Can you work these out from the model? Positions are in its coordinate system, mm. A direction names the side the tool comes from. Give positions to 0.01 mm unless a question says otherwise; leave off trailing zeros. Write each loop counter-clockwise with the first axis right and the second up, starting at its lowest first coordinate (ties: lowest second). Pieces come first, ordered by that corner, then holes.
```python
from build123d import *

# Parameters (mm, degrees)
SKETCH1_W           = 85
SKETCH1_H           = 85
SKETCH1_R           = 26
BOSS_EXTRUDE1_DEPTH = 10
SKETCH2_R           = 1.75
CUT_EXTRUDE1_DEPTH  = 11
SKETCH3_W           = 85
SKETCH3_H           = 85
SKETCH3_W_2         = 82
SKETCH3_H_2         = 82
BOSS_EXTRUDE2_DEPTH = 50
SKETCH4_R           = 1.6
CUT_EXTRUDE2_DEPTH  = 86
SKETCH5_R           = 40
SKETCH5_R_2         = 38.5
CUT_EXTRUDE3_DEPTH  = 7


with BuildPart() as part:
    # Sketch1 → Boss-Extrude1 (new body)
    with BuildSketch(Plane(origin=(0, 0, 0), x_dir=(1, 0, 0), z_dir=(0, 1, 0))):
        Rectangle(SKETCH1_W, SKETCH1_H)
        Circle(SKETCH1_R, mode=Mode.SUBTRACT)
    extrude(amount=BOSS_EXTRUDE1_DEPTH)

    # Sketch2 → Cut-Extrude1 (cut, through all)
    with BuildSketch(Plane(origin=(0, 10, 0), x_dir=(1, 0, 0), z_dir=(0, 1, 0))):
        with Locations((22.628070081, 22.628070081)):
            Circle(SKETCH2_R)
        with Locations((-22.626763915, 22.626763915)):
            Circle(SKETCH2_R)
        with Locations((-22.626763915, -22.626763915)):
            Circle(SKETCH2_R)
        with Locations((22.628070081, -22.628070081)):
            Circle(SKETCH2_R)
    extrude(amount=-CUT_EXTRUDE1_DEPTH, mode=Mode.SUBTRACT)

    # Sketch3 → Boss-Extrude2 (add)
    with BuildSketch(Plane(origin=(0, 0, 0), x_dir=(-1, 0, 0), z_dir=(0, -1, 0))):
        Rectangle(SKETCH3_W, SKETCH3_H)
        Rectangle(SKETCH3_W_2, SKETCH3_H_2, mode=Mode.SUBTRACT)
    extrude(amount=BOSS_EXTRUDE2_DEPTH)

    # Sketch4 → Cut-Extrude2 (cut, through all)
    with BuildSketch(Plane.ZY.offset(42.5)):
        with Locations((0, -18.6)):
            Circle(SKETCH4_R)
    extrude(amount=-CUT_EXTRUDE2_DEPTH, mode=Mode.SUBTRACT)

    # Sketch5 → Cut-Extrude3 (cut)
    with BuildSketch(Plane(origin=(0, 10, 0), x_dir=(1, 0, 0), z_dir=(0, 1, 0))):
        Circle(SKETCH5_R)
        Circle(SKETCH5_R_2, mode=Mode.SUBTRACT)
    extrude(amount=-CUT_EXTRUDE3_DEPTH, mode=Mode.SUBTRACT)


solid = part.part
```
1) Suppose I cut it at A-A on z = 0. Write out the boundary of the cut face in (x, y), plus the area to 3 significant figures.
Values follow:
outline: (-42.5, -50) - (-41, -50) - (-41, -20.2) - (-42.5, -20.2) - close; (-42.5, -17) - (-41, -17) - (-41, 0) - (-26, 0) - (-26, 10) - (-38.5, 10) - (-38.5, 3) - (-40, 3) - (-40, 10) - (-42.5, 10) - close; (26, 0) - (41, 0) - (41, -17) - (42.5, -17) - (42.5, 10) - (40, 10) - (40, 3) - (38.5, 3) - (38.5, 10) - (26, 10) - close; (41, -50) - (42.5, -50) - (42.5, -20.2) - (41, -20.2) - close
area: 449 mm2
2) If we mould it in two halves opening along X, with no side actions, what happens to faces 4 (the face through (42.5, -26, 1)), 5 (the face through (-20.633, 4.93, 15.821)), 6 (the face through (-41.76, -20.16, -0.35))? For each: +X half, -X half, draft (parallel to the pull), parting line (faces both ways), or undercut.
Values follow:
face 4: +X half
face 5: undercut
face 6: draft
3) Please list where these lines run through material, in increasing order: L1, parallel to X at y = 6, z = 0; L2, parallel to Z at x = 22.5, y = -36; L3, parallel to Y at x = -41.45, z = 0.
Values follow:
L1: x = -42.5 to -40, -38.5 to -26, 26 to 38.5, 40 to 42.5
L2: z = -42.5 to -41, 41 to 42.5
L3: y = -50 to -20.2, -17 to 10
4) For pin 1 Ø3 at (x, z) = (-24, -18.5) entering from -Y, with a flat end and sliding along its axis, tell me the tip position at first contact or that it passes through.
Values follow:
pin 1: stops at y = 0
5) Suppose I cut it at D-D on z = -16. Write out the boundary of the cut face in (x, y).
Values follow:
outline: (-42.5, -50) - (-41, -50) - (-41, 0) - (-20.49, 0) - (-20.49, 10) - (-35.02, 10) - (-35.02, 3) - (-36.66, 3) - (-36.66, 10) - (-42.5, 10) - close; (20.49, 0) - (41, 0) - (41, -50) - (42.5, -50) - (42.5, 10) - (36.66, 10) - (36.66, 3) - (35.02, 3) - (35.02, 10) - (20.49, 10) - close
6) Suppose I cut it at C-C on x = 0. Write out the boundary of the cut face in (y, z).
Values follow:
outline: (-50, -42.5) - (10, -42.5) - (10, -40) - (3, -40) - (3, -38.5) - (10, -38.5) - (10, -26) - (0, -26) - (0, -41) - (-50, -41) - close; (-50, 41) - (0, 41) - (0, 26) - (10, 26) - (10, 38.5) - (3, 38.5) - (3, 40) - (10, 40) - (10, 42.5) - (-50, 42.5) - close
7) For faces 1 (the face through (1, -25, -41)), 2 (the face through (-21, 3, -33)), 3 (the face through (-13, 10, -38)), which set-ups out of +Z, -Z, +X, -X, +Y, -Y let a thin tool reach every point of the face, with its end or its side?
Values follow:
face 1: -Y
face 2: +Y
face 3: +Z, -Z, +X, -X, +Y
8) Suppose I cut it at B-B on y = -24.5. Write out the boundary of the cut face in (x, z).
Values follow:
outline: (-42.5, -42.5) - (42.5, -42.5) - (42.5, 42.5) - (-42.5, 42.5) - close; hole (-41, -41) - (41, -41) - (41, 41) - (-41, 41) - close
